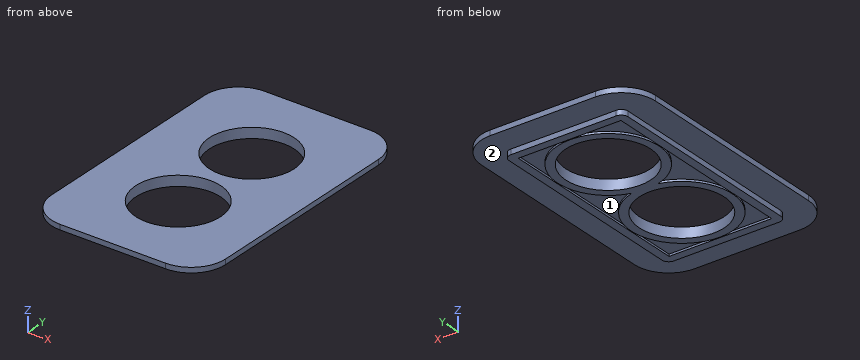
```python
from build123d import *

# Parameters (mm, degrees)
F0_W     = 34.7
F0_H     = 63.2
F0_R     = 12.35
F1_DEPTH = 3
F2_R     = 2
F3_T     = -2.4
F4_R     = 12.35
F5_DEPTH = 1.5


with BuildPart() as f1:
    # F0 (on Top) → F1 (new body)
    with BuildSketch(Plane.XY):
        Rectangle(F0_W, F0_H)
        with Locations((0, -14.25)):
            Circle(F0_R, mode=Mode.SUBTRACT)
        with Locations((0, 14.25)):
            Circle(F0_R, mode=Mode.SUBTRACT)
    extrude(amount=F1_DEPTH)

    # F2
    f2_edges = [f1.edges().sort_by_distance(p)[0] for p in [
        (-17.35, 31.6, 1.5),
        (-17.35, -31.6, 1.5),
        (17.35, -31.6, 1.5),
        (17.35, 31.6, 1.5),
    ]]
    fillet(f2_edges, radius=F2_R)

    # F3
    f3_openings = [f1.faces().sort_by_distance(p)[0] for p in [
        (0, 0, 0),
    ]]
    offset(amount=F3_T, openings=f3_openings)

    # F4 (on face) → F5 (join)
    with BuildSketch(Plane.XY.offset(3)):
        with BuildLine():
            Line((25.35, -29.6), (25.35, 29.6))
            ThreePointArc((25.35, 29.6), (22.4210678119, 36.6710678119), (15.35, 39.6))
            Line((15.35, 39.6), (-15.35, 39.6))
            ThreePointArc((-15.35, 39.6), (-22.4210678119, 36.6710678119), (-25.35, 29.6))
            Line((-25.35, 29.6), (-25.35, -29.6))
            ThreePointArc((-25.35, -29.6), (-22.4210678119, -36.6710678119), (-15.35, -39.6))
            Line((-15.35, -39.6), (15.35, -39.6))
            ThreePointArc((15.35, -39.6), (22.4210678119, -36.6710678119), (25.35, -29.6))
        make_face()
        with Locations((0, -14.25)):
            Circle(F4_R, mode=Mode.SUBTRACT)
        with Locations((0, 14.25)):
            Circle(F4_R, mode=Mode.SUBTRACT)
    extrude(amount=-F5_DEPTH)


solid = f1.part
```
Part model, mm, in its own coordinate system. Face numbers are marked on the shaded views. Coordinates: 2 decimals unless noted, no trailing zeros. Loops run counter-clockwise (first coordinate to the right, second up) from the corner with the lowest first, then second, coordinate; pieces in that order, holes last. Notation, with made-up numbers: (17.25, 15) - (25.25, 15) arc R20 ccw to (25.25, 36) - close; hole circle Ø6 at (-11, 87). An arc over 180 degrees is marked (long way). Write item = value, one per line. Start each with the question number.
Item 1: Cut at C-C, the plane z = 1.05. Give the cut face in (x, y), and give its area (3 significant figures).
Item 2: Cut at A-A, the plane y = -14.25. Give the cut face in (x, z), and give its area (3 significant figures).
Item 3: Cut at D-D, the plane y = -4.5. Give the cut face in (x, z), and give its area (3 significant figures).
Item 4: Wall check: L1, parallel to Y at x = 0, z = 0.8; L2, parallel to Y at x = 0, z = 1.6; L3, parallel to Y at x = 8, z = 0.4. Give the ranges that are in metal, low to high. Write a range as from..to.
Item 5: Flat gauge pins, fed straight in: pin 1 Ø0.7 at (y, z) = (-0.5, 0.5) entering from +X; pin 2 Ø1.2 at (x, z) = (-7, 1) entering from -Y; pin 3 Ø0.5 at (x, z) = (-6.5, 0.5) entering from +Y; pin 4 Ø0.8 at (y, z) = (-11, 0.5) entering from -X. Where does each tip first touch, or does it go through?
Item 6: Mould opens along X. For the marked faces 1 and 2 say: released by +X, released by -X, zero draft, split by the parting line, or undercut.
Item 7: Cut at B-B, the plane x = 0. Give the cut face in (y, z).
The answers:
q1.outline = (-17.35, -29.6) arc R2 ccw to (-15.35, -31.6) - (15.35, -31.6) arc R2 ccw to (17.35, -29.6) - (17.35, 29.6) arc R2 ccw to (15.35, 31.6) - (-15.35, 31.6) arc R2 ccw to (-17.35, 29.6) - close; hole circle Ø24.7 at (0, -14.25); hole circle Ø24.7 at (0, 14.25)
q1.area = 1,230 mm2
q2.outline = (-25.35, 1.5) - (-17.35, 1.5) - (-17.35, 0) - (-14.95, 0) - (-14.95, 0.6) - (-14.75, 0.6) - (-14.75, 0) - (-12.35, 0) - (-12.35, 3) - (-25.35, 3) - close; (12.35, 0) - (14.75, 0) - (14.75, 0.6) - (14.95, 0.6) - (14.95, 0) - (17.35, 0) - (17.35, 1.5) - (25.35, 1.5) - (25.35, 3) - (12.35, 3) - close
q2.area = 53.8 mm2
q3.outline = (-25.35, 1.5) - (-17.35, 1.5) - (-17.35, 0) - (-14.95, 0) - (-14.95, 0.6) - (-11.07, 0.6) - (-11.07, 0) - (-7.58, 0) - (-7.58, 3) - (-25.35, 3) - close; (7.58, 0) - (11.07, 0) - (11.07, 0.6) - (14.95, 0.6) - (14.95, 0) - (17.35, 0) - (17.35, 1.5) - (25.35, 1.5) - (25.35, 3) - (7.58, 3) - close
q3.area = 78.0 mm2
q4.L1 = -31.6..-26.6, -1.9..1.9, 26.6..31.6
q4.L2 = -39.6..-26.6, -1.9..1.9, 26.6..39.6
q4.L3 = -31.6..-29.2, -26.64..-23.66, -4.84..-1.86, 1.86..4.84, 23.66..26.64, 29.2..31.6
q5.pin_1 = 17.35
q5.pin_2 = -39.6
q5.pin_3 = 31.6
q5.pin_4 = -17.35
q6.face_1 = undercut
q6.face_2 = zero draft
q7.outline = (-39.6, 1.5) - (-31.6, 1.5) - (-31.6, 0) - (-29.2, 0) - (-29.2, 0.6) - (-29, 0.6) - (-29, 0) - (-26.6, 0) - (-26.6, 3) - (-39.6, 3) - close; (-1.9, 0) - (1.9, 0) - (1.9, 3) - (-1.9, 3) - close; (26.6, 0) - (29, 0) - (29, 0.6) - (29.2, 0.6) - (29.2, 0) - (31.6, 0) - (31.6, 1.5) - (39.6, 1.5) - (39.6, 3) - (26.6, 3) - close
